Verification items for this drawing (mm, ordinates from the low corner). Round coordinates to 2 decimals unless told otherwise and drop trailing zeros. Write each loop counter-clockwise with the first axis right and the second up, starting at its lowest first coordinate (ties: lowest second). Pieces come first, ordered by that corner, then holes.
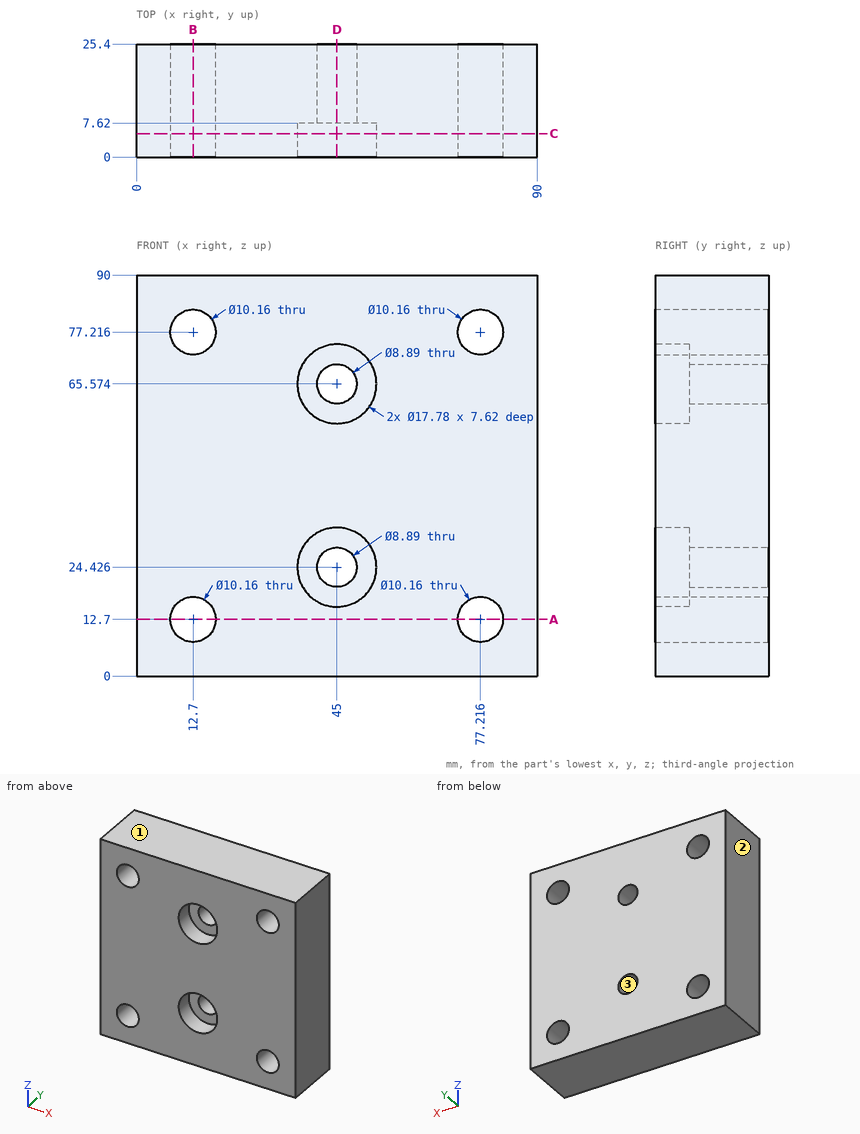
1. Scan lines: line 1 along X through (y, z) = (19, 12.5); line 2 along Z through (x, y) = (12.7, 5); line 3 along Z through (x, y) = (45, 15). Record each from-to range of solid material in increasing order.
2. Section check A-A (z = 12.7). Record the cut outline in (x, y), plus the area to 3 significant figures.
3. Section check C-C (y = 5.25). Record the cut outline in (x, z).
4. Depth check by flat-ended pin: pin 1 Ø14 at (x, z) = (45, 65.574) entering from -Y. Enter the tip coordinate at first touch or a pass-through.
5. Section check D-D (x = 45). Record the cut outline in (y, z), plus the area to 3 significant figures.
6. Release check for a two-part mould opening along Z. For the marked faces 1, 2 and 3 record: +Z half, -Z half, draft (parallel to the pull), parting line (faces both ways), or undercut.
7. Section check B-B (x = 12.7). Record the cut outline in (y, z).
Results below:
1. line 1: x = 0 to 7.62, 17.78 to 72.14, 82.29 to 90
1. line 2: z = 0 to 7.62, 17.78 to 72.14, 82.3 to 90
1. line 3: z = 0 to 19.98, 28.87 to 61.13, 70.02 to 90
2. outline: (0, 0) - (7.62, 0) - (7.62, 25.4) - (0, 25.4) - close; (17.78, 0) - (72.14, 0) - (72.14, 25.4) - (17.78, 25.4) - close; (82.3, 0) - (90, 0) - (90, 25.4) - (82.3, 25.4) - close
2. area: 1,770 mm2
3. outline: (0, 0) - (90, 0) - (90, 90) - (0, 90) - close; hole circle Ø10.16 at (12.7, 12.7); hole circle Ø10.16 at (12.7, 77.22); hole circle Ø17.78 at (45, 24.43); hole circle Ø17.78 at (45, 65.57); hole circle Ø10.16 at (77.22, 12.7); hole circle Ø10.16 at (77.22, 77.22)
4. pin 1: stops at y = 7.62
5. outline: (0, 0) - (25.4, 0) - (25.4, 19.98) - (7.62, 19.98) - (7.62, 15.54) - (0, 15.54) - close; (0, 33.32) - (7.62, 33.32) - (7.62, 28.87) - (25.4, 28.87) - (25.4, 61.13) - (7.62, 61.13) - (7.62, 56.68) - (0, 56.68) - close; (0, 74.46) - (7.62, 74.46) - (7.62, 70.02) - (25.4, 70.02) - (25.4, 90) - (0, 90) - close
5. area: 1,700 mm2
6. face 1: +Z half
6. face 2: draft
6. face 3: undercut
7. outline: (0, 0) - (25.4, 0) - (25.4, 7.62) - (0, 7.62) - close; (0, 17.78) - (25.4, 17.78) - (25.4, 72.14) - (0, 72.14) - close; (0, 82.3) - (25.4, 82.3) - (25.4, 90) - (0, 90) - close
